from build123d import *

# Parameters (mm, degrees)
F0_R     = 13
F0_R_2   = 10.5
F1_DEPTH = 5
F0_R_3   = 2.1
F2_DEPTH = 5
F3_SIZE2 = 2.7
F3_SIZE  = 2.7


with BuildPart() as f1:
    # F0 (on Front) → F1 (new body)
    with BuildSketch(Plane.XZ):
        with Locations((-16.9531982392, -2.1669319831)):
            Circle(F0_R)
        with Locations((-16.9531982392, -2.1669319831)):
            Circle(F0_R_2, mode=Mode.SUBTRACT)
    extrude(amount=F1_DEPTH)

    # F0 (on Front) → F2 (join)
    with BuildSketch(Plane.XZ):
        with Locations((-16.9531982392, -2.1669319831)):
            Circle(F0_R)
        with Locations((-16.9531982392, -2.1669319831)):
            Circle(F0_R_2, mode=Mode.SUBTRACT)
        with Locations((-16.9531982392, -2.1669319831)):
            Circle(F0_R_2)
        with Locations((-16.9531982392, -2.1669319831)):
            Circle(F0_R_3, mode=Mode.SUBTRACT)
    extrude(amount=-F2_DEPTH)

    # F3
    f3_edges = [f1.edges().sort_by_distance(p)[0] for p in [
        (-19.053198, 0, -2.166932),
    ]]
    chamfer(f3_edges, length=F3_SIZE, length2=F3_SIZE2)


solid = f1.part
Part model, mm, in its own coordinate system. A direction names the side the tool comes from. Round coordinates to 2 decimals unless told otherwise and drop trailing zeros. Write each loop counter-clockwise with the first axis right and the second up, starting at its lowest first coordinate (ties: lowest second). Pieces come first, ordered by that corner, then holes. Notation, with made-up numbers: M 70,-26 L 126,-26 A28 cw 126,7 Z; hole C -30,47.5 d9. An arc over 180 degrees is marked long. Return JSON: item names as keys, results as strings. Group by question number.
(1) Saw through at A-A on z = 5.25. Write the cut outline in (x, y), then the cut area to 3 significant figures.
(2) Which spindle directions (+Z, -Z, +X, -X, +Y, -Y) get a long thin tool onto all of the face, cutting with end or side? Do faces 4 (the face through (-6.94, -2.46, 0.99)), 5 (the face through (-18.62, 3.834, -3.445)). Say none if no direction does.
(3) Saw through at B-B on x = -24.5. Write the cut outline in (y, z).
(4) Two-plate mould, pull along Z, no slides. Class faces 1 (the face through (-15, 0, -7)), 2 (the face through (-4.554, -0.07, 1.738)), 3 (the face through (-14, 5, -2)): +Z half, -Z half, draft (parallel to the pull), parting line (faces both ways), or undercut.
(5) Saw through at D-D on y = 2.25. Write the cut outline in (x, z), then the cut area to 4 significant figures.
(6) Saw through at C-C on y = -0.5. Write the cut outline in (x, z), then the cut area to 3 significant figures.
(7) Drill centre lines: probe 1 along Z at (x, y) = (-17, -2); probe 2 along X at (y, z) = (-4, -2.25); probe 3 along Y at (x, z) = (-24.75, -8). Where is each one in solid material? Low to high.
(8) Pin check, flat tips, straight feed: pin 1 Ø5 at (x, z) = (-20.5, -1) entering from -Y; pin 2 Ø2 at (y, z) = (-1, -4.5) entering from +X; pin 3 Ø6.5 at (x, z) = (-15.5, -2.5) entering from -Y. Stop position of each tip, or through.
Returned:
{
 "1": {"outline": "M -27.63,-5 L -24.39,-5 L -24.39,0 L -9.52,0 L -9.52,-5 L -6.28,-5 L -6.28,5 L -27.63,5 Z", "area": "139 mm²"},
 "2": {"face 4": "-Y", "face 5": "+Y, -Y"},
 "3": {"outline": "M -5,-12.75 L 5,-12.75 L 5,8.42 L -5,8.42 L -5,5.13 L 0,5.13 L 0,-9.47 L -5,-9.47 Z"},
 "4": {"face 1": "undercut", "face 2": "parting line", "face 3": "draft"},
 "5": {"outline": "C -16.95,-2.17 d26; hole C -16.95,-2.17 d5.1", "area": "510.5 mm²"},
 "6": {"outline": "C -16.95,-2.17 d26; hole C -16.95,-2.17 d21", "area": "185 mm²"},
 "7": {"probe 1": "-15.17 to -12.67, 8.33 to 10.83", "probe 2": "-29.95 to -27.45, -6.45 to -3.95", "probe 3": "0 to 5"},
 "8": {"pin 1": "y = 0", "pin 2": "x = -4.02", "pin 3": "y = 0.06"}
}
